Can you work these out from the model? Positions are in its coordinate system, mm. Give positions to 0.01 mm unless a question says otherwise; leave off trailing zeros. Order: outer loops, then holes, each group sorted by start corner. A loop starts at its lowest first (then second) coordinate and runs counter-clockwise, first axis right, second up. Notation, with made-up numbers: (9.25, 32) - (21.25, 32) arc R17 ccw to (21.25, 42) - close; hole circle Ø9 at (13.5, -20.75). An arc over 180 degrees is marked (long way). Return JSON: item names as keys, results as strings.
```python
from build123d import *

# Parameters (mm, degrees)
F0_R     = 1.5875
F0_R_2   = 0.79375
F1_DEPTH = 3.175


with BuildPart() as f1:
    # F0 (on Front) → F1 (new body)
    with BuildSketch(Plane.XZ):
        with BuildLine():
            ThreePointArc((1.419532, 43.416747), (-3.070596, 41.556875), (-4.930468, 37.066747))
            Line((-4.930468, 37.066747), (-4.930468, -139.158453))
            ThreePointArc((-4.930468, -139.158453), (-3.070596, -143.648581), (1.419532, -145.508453))
            ThreePointArc((1.419532, -145.508453), (5.90966, -143.648581), (7.769532, -139.158453))
            Line((7.769532, -139.158453), (7.769532, 37.066747))
            ThreePointArc((7.769532, 37.066747), (5.90966, 41.556875), (1.419532, 43.416747))
        make_face()
        with Locations((1.419532, -142.333453)):
            Circle(F0_R, mode=Mode.SUBTRACT)
        with Locations((1.419532, 40.241747)):
            Circle(F0_R_2, mode=Mode.SUBTRACT)
    extrude(amount=F1_DEPTH)


solid = f1.part
```
1. Suppose I cut it at B-B (x = 6). List the corners of the cut face in (y, z) for me (3 decimals), plus the area to 3 significant figures.
Checks:
{"outline": "(-3.175, -143.556) - (0, -143.556) - (0, 41.465) - (-3.175, 41.465) - close", "area": "587 mm^2"}
2. If I drill on L1, parallel to Z at x = 1.75, y = -2; L2, parallel to Z at x = -2, y = -1.5; L3, parallel to Z at x = -2.25, y = -1.7, over which ranges is the centre line in solid material (lowest first)? Write a range as [from, to].
Checks:
{"L1": "[-145.5, -143.89], [-140.78, 39.52], [40.96, 43.41]", "L2": "[-144.51, 42.42]", "L3": "[-144.34, 42.25]"}
3. Thinking about a two-plate mould opening in X: for faces 1 (the face through (2.273, -1.565, -140.995)), 2 (the face through (7.77, -2, -52)), 3 (the face through (1, -3.175, -50)), which applies, +X half, -X half, draft (parallel to the pull), parting line (faces both ways), or undercut?
Checks:
{"face 1": "undercut", "face 2": "+X half", "face 3": "draft"}
4. Suppose I cut it at A-A (y = -0.5). State how many separate pieces and enclosed holes the cut face has, plus the area to 3 significant figures.
Checks:
{"separate pieces": "1", "enclosed holes": "2", "area": "2,350 mm^2"}
